Work out the finished part from the listing and answer in its coordinate system (mm). Give positions to 0.01 mm unless a question says otherwise; leave off trailing zeros. Write each loop counter-clockwise with the first axis right and the second up, starting at its lowest first coordinate (ties: lowest second). Pieces come first, ordered by that corner, then holes. Notation, with made-up numbers: (-19.5, 86.5) - (10.5, 86.5) arc R13 ccw to (10.5, 100.5) - close; hole circle Ø1 at (55, 50.5). An arc over 180 degrees is marked (long way). Write each question's results on one line, items separated by ' | '. Start each with the question number.
from build123d import *

# Parameters (mm, degrees)
SKETCH1_R           = 4
SKETCH1_R_2         = 3.4
SKETCH1_R_3         = 11
BOSS_EXTRUDE3_DEPTH = 5
SKETCH2_R           = 2.5
CUT_EXTRUDE1_DEPTH  = 10


with BuildPart() as part:
    # Sketch1 → Boss-Extrude3 (new body)
    with BuildSketch(Plane.XY):
        with BuildLine():
            Line((0, 25), (180, 25))
            ThreePointArc((180, 25), (205, 0), (180, -25))
            Line((180, -25), (0, -25))
            ThreePointArc((0, -25), (-25, 0), (0, 25))
        make_face()
        Circle(SKETCH1_R, mode=Mode.SUBTRACT)
        with Locations((-16, 0)):
            Circle(SKETCH1_R_2, mode=Mode.SUBTRACT)
        with Locations((16, 0)):
            Circle(SKETCH1_R_2, mode=Mode.SUBTRACT)
        with Locations((180, 0)):
            Circle(SKETCH1_R_3, mode=Mode.SUBTRACT)
    extrude(amount=BOSS_EXTRUDE3_DEPTH)

    # Sketch2 → Cut-Extrude1 (cut)
    with BuildSketch(Plane.XY.offset(5)):
        with Locations((90, 15)):
            Circle(SKETCH2_R)
        with Locations((90, -15)):
            Circle(SKETCH2_R)
    extrude(amount=-CUT_EXTRUDE1_DEPTH, mode=Mode.SUBTRACT)


solid = part.part
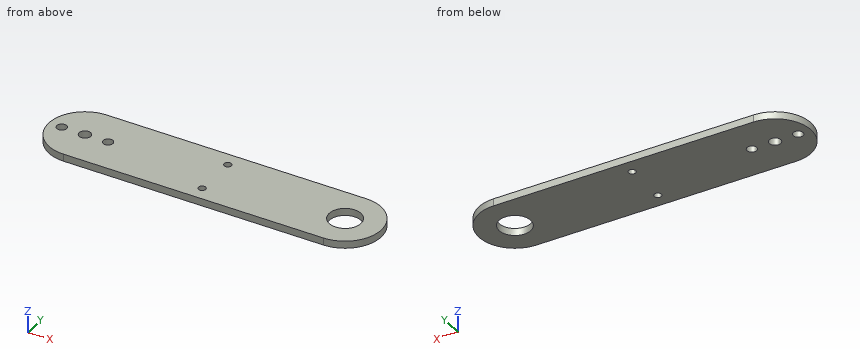
Q1. A cutting plane is placed at A-A, the plane y = 0. Write down the section's boundary in (x, z), and give its area (3 significant figures).
Q2. Consider L1, parallel to Y at x = 90, z = 1.8; L2, parallel to X at y = -2.5, z = 4.15; L3, parallel to X at y = -3, z = 0.65. Determine where each line is inside the solid, lowest interval first.
Q3. A cutting plane is placed at C-C, the plane z = 4.2. Write down the section's boundary in (x, y), and give its area (3 significant figures).
Q4. A cutting plane is placed at D-D, the plane y = -15. Write down the section's boundary in (x, z), and give its area (4 significant figures).
Q5. A cutting plane is placed at B-B, the plane x = 16. Write down the section's boundary in (y, z), and give its area (3 significant figures).
Result:
1) outline: (-25, 0) - (-19.4, 0) - (-19.4, 5) - (-25, 5) - close; (-12.6, 0) - (-4, 0) - (-4, 5) - (-12.6, 5) - close; (4, 0) - (12.6, 0) - (12.6, 5) - (4, 5) - close; (19.4, 0) - (169, 0) - (169, 5) - (19.4, 5) - close; (191, 0) - (205, 0) - (205, 5) - (191, 5) - close | area: 932 mm2
2) L1: y = -25 to -17.5, -12.5 to 12.5, 17.5 to 25 | L2: x = -24.87 to -18.3, -13.7 to -3.12, 3.12 to 13.7, 18.3 to 169.29, 190.71 to 204.87 | L3: x = -24.82 to -17.6, -14.4 to -2.65, 2.65 to 14.4, 17.6 to 169.42, 190.58 to 204.82
3) outline: (0, -25) - (180, -25) arc R25 ccw to (180, 25) - (0, 25) arc R25 ccw to start; hole circle Ø6.8 at (-16, 0); hole circle Ø8 at (0, 0); hole circle Ø6.8 at (16, 0); hole circle Ø5 at (90, -15); hole circle Ø5 at (90, 15); hole circle Ø22 at (180, 0) | area: 10,400 mm2
4) outline: (-20, 0) - (87.5, 0) - (87.5, 5) - (-20, 5) - close; (92.5, 0) - (200, 0) - (200, 5) - (92.5, 5) - close | area: 1,075 mm2
5) outline: (-25, 0) - (-3.4, 0) - (-3.4, 5) - (-25, 5) - close; (3.4, 0) - (25, 0) - (25, 5) - (3.4, 5) - close | area: 216 mm2
